from build123d import *

# Parameters (mm, degrees)
F0_W     = 131.769553
F0_H     = 77.441782
F1_DEPTH = 25.4
F2_R     = 12.7
F3_DEPTH = 25.4
F4_W     = 25.4
F4_H     = 25.4
F5_DEPTH = 25.4


with BuildPart() as f1:
    # F0 (on Front) → F1 (new body)
    with BuildSketch(Plane.XZ):
        with Locations((10.569222, 0.197556)):
            Rectangle(F0_W, F0_H)
    extrude(amount=F1_DEPTH)

    # F2 (on Front) → F3 (cut)
    with BuildSketch(Plane.XZ):
        with Locations((56.035224, -11.260667)):
            Circle(F2_R)
    extrude(amount=F3_DEPTH, mode=Mode.SUBTRACT)

    # F4 (on face) → F5 (cut)
    with BuildSketch(Plane.XZ.offset(25.4)):
        with Locations((-20.277668, 18.034001)):
            Rectangle(F4_W, F4_H)
    extrude(amount=-F5_DEPTH, mode=Mode.SUBTRACT)


solid = f1.part
Could you check a few things on this model? Use its own coordinates, in mm. A direction names the side the tool comes from. Give positions to 0.01 mm unless a question says otherwise; leave off trailing zeros. Order: outer loops, then holes, each group sorted by start corner. A loop starts at its lowest first (then second) coordinate and runs counter-clockwise, first axis right, second up.
1. Suppose I cut it at B-B (z = -15). Write out the boundary of the cut face in (x, y), plus the area to 3 significant figures.
Answers below:
outline: (-55.32, -25.4) - (43.9, -25.4) - (43.9, 0) - (-55.32, 0) - close; (68.17, -25.4) - (76.45, -25.4) - (76.45, 0) - (68.17, 0) - close
area: 2,730 mm2
2. Suppose I cut it at A-A (x = -19). Write out the boundary of the cut face in (y, z).
Answers below:
outline: (-25.4, -38.52) - (0, -38.52) - (0, 5.33) - (-25.4, 5.33) - close; (-25.4, 30.73) - (0, 30.73) - (0, 38.92) - (-25.4, 38.92) - close
3. Which directions (+Z, -Z, +X, -X, +Y, -Y) give clear straight access to the entire face, cutting with the end or side of a thin tool? Please do faces 1 (the flat face through (10, -25.4, 1)), 2 (the flat face through (-20, -13, 5.334)).
Answers below:
face 1: +Z, -Z, +X, -X, -Y
face 2: +Y, -Y
4. I need wall thicknesses on L1, parallel to X at y = -9, z = 30.5; L2, parallel to Z at x = -26, y = -20; L3, parallel to Z at x = 56, y = -23.75. Which ranges of each line are inside material? Lowest first, please.
Answers below:
L1: x = -55.32 to -32.98, -7.58 to 76.45
L2: z = -38.52 to 5.33, 30.73 to 38.92
L3: z = -38.52 to -23.96, 1.44 to 38.92
5. Suppose I cut it at C-C (y = -8.75). Write out the boundary of the cut face in (x, z), plus the area to 3 significant figures.
Answers below:
outline: (-55.32, -38.52) - (76.45, -38.52) - (76.45, 38.92) - (-55.32, 38.92) - close; hole (-32.98, 5.33) - (-7.58, 5.33) - (-7.58, 30.73) - (-32.98, 30.73) - close; hole circle Ø25.4 at (56.04, -11.26)
area: 9,050 mm2
6. Thinking about a two-plate mould opening in X: for faces 3 (the flat face through (10, 0, 1)), 4 (the flat face through (76.454, -13, 0)), 5 (the flat face through (-20, -13, 30.734)), which applies, +X half, -X half, draft (parallel to the pull), parting line (faces both ways), or undercut?
Answers below:
face 3: draft
face 4: +X half
face 5: undercut
